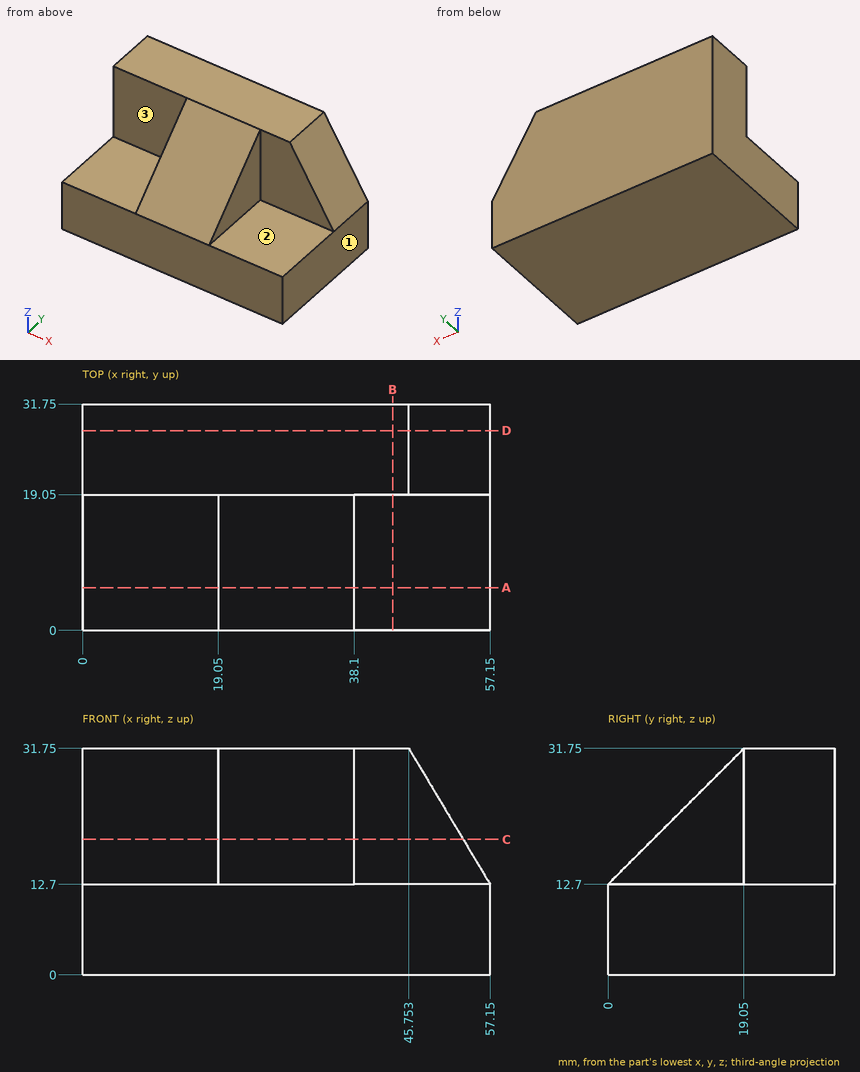
The drawing under review shows one solid part. Ordinate dimensions are in mm from its lowest x, y, z. A direction names the side the tool comes from. Round coordinates to 2 decimals unless told otherwise and drop trailing zeros. Order: outer loops, then holes, each group sorted by start corner. A loop starts at its lowest first (then second) coordinate and runs counter-clockwise, first axis right, second up. Notation, with made-up numbers: (25, 80.25) - (55, 80.25) arc R36 ccw to (55, 117.25) - close; hole circle Ø2 at (3.5, 12.5). An arc over 180 degrees is marked (long way). Return JSON: item names as keys, results as strings.
Q1. Consider section D-D on y = 28. Write out the cut boundary in (x, z), plus the area to 3 significant figures.
Computed values:
{"outline": "(0, 0) - (57.15, 0) - (57.15, 12.7) - (45.75, 31.75) - (0, 31.75) - close", "area": "1,710 mm2"}
Q2. Wall thickness on L1, parallel to Y at x = 6, z = 18; L2, parallel to Z at x = 19, y = 18; L3, parallel to X at y = 18.5, z = 29: over which ranges is each line inside the solid? List them lowest first. Write a range as [from, to].
Computed values:
{"L1": "y = [19.05, 31.75]", "L2": "z = [0, 12.7]", "L3": "x = [19.05, 38.1]"}
Q3. Consider section C-C on z = 19. Write out the cut boundary in (x, y).
Computed values:
{"outline": "(0, 19.05) - (19.05, 19.05) - (19.05, 6.3) - (38.1, 6.3) - (38.1, 19.05) - (53.38, 19.05) - (53.38, 31.75) - (0, 31.75) - close"}
Q4. For pin 1 Ø6 at (x, y) = (8, 8) entering from +Z; pin 2 Ø1 at (y, z) = (13.5, 16) entering from -X; pin 3 Ø5.5 at (x, z) = (7, 26.5) entering from -Y; pin 4 Ø1.5 at (x, z) = (17.5, 3.5) entering from -Y, all flat-tipped, find the tip position at first contact; note any pin that passes through.
Computed values:
{"pin 1": "stops at z = 12.7", "pin 2": "stops at x = 19.05", "pin 3": "stops at y = 19.05", "pin 4": "stops at y = 0"}
Q5. Machinability: for the marked faces 1, 2 and 3, which of the approach directions +Z, -Z, +X, -X, +Y, -Y give a long, thin tool a straight path to every point of the face, cutting with its end or side? Answer none if there is none.
Computed values:
{"face 1": "+Z, -Z, +X, +Y, -Y", "face 2": "+Z, +X, -Y", "face 3": "+Z, -X, -Y"}
Q6. Consider section A-A on y = 6. Write out the cut boundary in (x, z), plus the area to 3 significant figures.
Computed values:
{"outline": "(0, 0) - (57.15, 0) - (57.15, 12.7) - (38.1, 12.7) - (38.1, 18.7) - (19.05, 18.7) - (19.05, 12.7) - (0, 12.7) - close", "area": "840 mm2"}
Q7. Consider section B-B on x = 43.5. Write out the cut boundary in (y, z), plus the area to 3 significant figures.
Computed values:
{"outline": "(0, 0) - (31.75, 0) - (31.75, 31.75) - (19.05, 31.75) - (19.05, 12.7) - (0, 12.7) - close", "area": "645 mm2"}
